```python
from build123d import *

# Parameters (mm, degrees)
BOSS_EXTRUDE2_DEPTH = 15


with BuildPart() as part:
    # Sketch2 → Boss-Extrude2 (new body)
    with BuildSketch(Plane(origin=(0, 0, 0), x_dir=(1, 0, 0), z_dir=(0, 1, 0))):
        with BuildLine():
            Line((-28.349494605, 21.964136687), (-17.349494605, 21.964136687))
            Line((-17.349494605, 21.964136687), (-17.349494605, 25.764136687))
            Line((-17.349494605, 25.764136687), (-28.349494605, 25.764136687))
            Line((-28.349494605, 25.764136687), (-28.349494605, 28.764136687))
            Line((-28.349494605, 28.764136687), (21.650505395, 28.764136687))
            Line((21.650505395, 28.764136687), (21.650505395, 25.764136687))
            Line((21.650505395, 25.764136687), (10.650505395, 25.764136687))
            Line((10.650505395, 25.764136687), (10.650505395, 21.964136687))
            Line((10.650505395, 21.964136687), (21.650505395, 21.964136687))
            Line((21.650505395, 21.964136687), (21.650505395, 18.957031621))
            Line((21.650505395, 18.957031621), (4.150505395, 18.957031621))
            Line((4.150505395, 18.957031621), (4.150505395, 10.957031621))
            ThreePointArc((4.150505395, 10.957031621), (-3.329004451, 3.529483044), (-10.847714263, 10.91734797))
            Line((-10.847714263, 10.91734797), (-6.026180838, 10.932389281))
            Line((-6.026180838, 10.932389281), (-4.222493535, 9.423226245))
            Line((-4.222493535, 9.423226245), (-4.222493535, 8.122210377))
            Line((-4.222493535, 8.122210377), (-6.025980027, 8.122210377))
            Line((-6.025980027, 8.122210377), (-6.025980027, 9.423279207))
            Line((-6.025980027, 9.423279207), (-9.437714366, 9.423279207))
            ThreePointArc((-9.437714366, 9.423279207), (-2.574965526, 4.779817175), (2.947813029, 10.957031621))
            Line((2.947813029, 10.957031621), (2.947813029, 18.957031621))
            Line((2.947813029, 18.957031621), (-28.349494605, 18.957031621))
            Line((-28.349494605, 18.957031621), (-28.349494605, 21.964136687))
        make_face()
    extrude(amount=BOSS_EXTRUDE2_DEPTH)


solid = part.part
```
Work out the finished part from the listing and answer in its coordinate system (mm). A direction names the side the tool comes from. Round coordinates to 2 decimals unless told otherwise and drop trailing zeros. Loops run counter-clockwise (first coordinate to the right, second up) from the corner with the lowest first, then second, coordinate; pieces in that order, holes last.
(1) The part is cut by section C-C, the plane z = -6.25. Give the vertices of the cut face in (x, y).
Computed values:
outline: (-9.13, 0) - (-7.45, 0) - (-7.45, 15) - (-9.13, 15) - close; (0.75, 0) - (2.43, 0) - (2.43, 15) - (0.75, 15) - close
(2) The part is cut by section D-D, the plane x = -8. Give the vertices of the cut face in (y, z), and give its area (3 significant figures).
Computed values:
outline: (0, -28.76) - (15, -28.76) - (15, -18.96) - (0, -18.96) - close; (0, -10.93) - (15, -10.93) - (15, -9.42) - (0, -9.42) - close; (0, -6.78) - (15, -6.78) - (15, -5.15) - (0, -5.15) - close
area: 194 mm2
(3) For faces 1 (the flat face through (-17.349, 7, -24)), 2 (the flat face through (16, 7, -21.964)), 3 (the flat face through (-5, 7, -8.122)), determine the directions among +Z, -Z, +X, -X, +Y, -Y from which every point of the face is accessible in a straight line to the end or side of a thin tool.
Computed values:
face 1: -X, +Y, -Y
face 2: +X, +Y, -Y
face 3: +Y, -Y
(4) Find the intervals of material crossed by L1, parallel to Z at x = 12, y = 7.25; L2, parallel to Z at x = -8, y = 10.25; L3, parallel to X at y = 12.5, z = -9.25, in increasing order.
Computed values:
L1: z = -28.76 to -25.76, -21.96 to -18.96
L2: z = -28.76 to -18.96, -10.93 to -9.42, -6.78 to -5.15
L3: x = -10.63 to -9.39, -6.03 to -4.22, 2.69 to 3.94
(5) The part is cut by section A-A, the plane x = 15. Give the vertices of the cut face in (y, z), and give its area (3 significant figures).
Computed values:
outline: (0, -28.76) - (15, -28.76) - (15, -25.76) - (0, -25.76) - close; (0, -21.96) - (15, -21.96) - (15, -18.96) - (0, -18.96) - close
area: 90.1 mm2
(6) The mould has two halves that part along X. Classify faces 4 (the flat face through (-8, 7, -9.423)), 5 (the flat face through (10.651, 7, -24)), 6 (the flat face through (-12, 7, -18.957)): pulls with the +X half, pulls with the -X half, needs draft (parallel to the pull), parting line crosses it, or undercut.
Computed values:
face 4: undercut
face 5: pulls with the +X half
face 6: needs draft
(7) The part is cut by section B-B, the plane y = 8.25. Give the vertices of the cut face in (x, z).
Computed values:
outline: (-28.35, -28.76) - (21.65, -28.76) - (21.65, -25.76) - (10.65, -25.76) - (10.65, -21.96) - (21.65, -21.96) - (21.65, -18.96) - (4.15, -18.96) - (4.15, -10.96) arc R7.5 ccw to (-10.85, -10.92) - (-6.03, -10.93) - (-4.22, -9.42) - (-4.22, -8.12) - (-6.03, -8.12) - (-6.03, -9.42) - (-9.44, -9.42) arc R6.3 cw to (2.95, -10.96) - (2.95, -18.96) - (-28.35, -18.96) - (-28.35, -21.96) - (-17.35, -21.96) - (-17.35, -25.76) - (-28.35, -25.76) - close
(8) Each of these flat-tipped pins is pushed along its axis until it touches: P1, Ø3, axis at y = 7.5, z = -25, coming from the +X side; P2, Ø1.1, axis at y = 9, z = -25, coming from the -X side; P3, Ø9, axis at x = 17.5, y = 9, coming from the +Z side; P4, Ø4.5, axis at x = -11.5, y = 7.5, coming from the +Z side. Where does it stop, or does it pass through?
Computed values:
P1: stops at x = 21.65
P2: stops at x = -17.35
P3: stops at z = -18.96
P4: stops at z = -6.4
